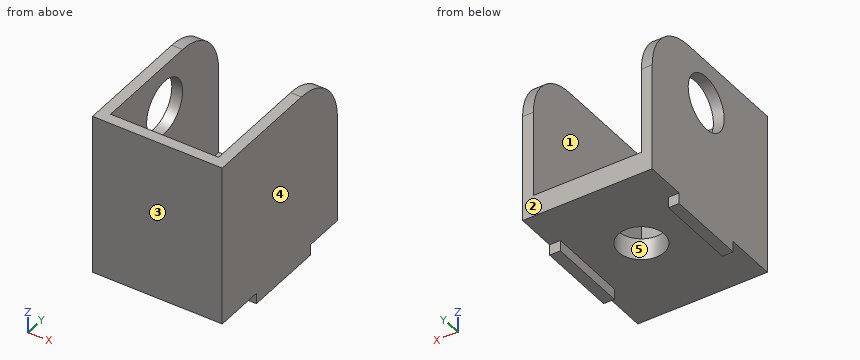
from build123d import *

# Parameters (mm, degrees)
SKETCH1_W           = 20
SKETCH1_H           = 30
SKETCH1_R           = 4.25
BOSS_EXTRUDE1_DEPTH = 4
SKETCH2_W           = 20
SKETCH2_H           = 30
BOSS_EXTRUDE2_DEPTH = 2
SKETCH4_R           = 5
BOSS_EXTRUDE3_DEPTH = 2
BOSS_EXTRUDE4_START = 2
BOSS_EXTRUDE4_DEPTH = 2
SKETCH6_W           = 2
SKETCH6_H           = 15
BOSS_EXTRUDE5_DEPTH = 2


with BuildPart() as part:
    # Sketch1 → Boss-Extrude1 (new body)
    with BuildSketch(Plane.XY):
        Rectangle(SKETCH1_W, SKETCH1_H)
        Circle(SKETCH1_R, mode=Mode.SUBTRACT)
    extrude(amount=BOSS_EXTRUDE1_DEPTH)

    # Sketch2 → Boss-Extrude2 (add)
    with BuildSketch(Plane(origin=(0, -15, 0), x_dir=(-1, 0, 0), z_dir=(0, -1, 0))):
        with Locations((0, -15)):
            Rectangle(SKETCH2_W, SKETCH2_H)
    extrude(amount=BOSS_EXTRUDE2_DEPTH)

    # Sketch4 → Boss-Extrude3 (add)
    with BuildSketch(Plane.ZY.offset(10)):
        with BuildLine():
            Line((0, 15), (20, 15))
            ThreePointArc((20, 15), (27.071067812, 12.071067812), (30, 5))
            Line((30, 5), (30, -17))
            Line((30, -17), (0, -17))
            Line((0, -17), (0, 15))
        make_face()
        with Locations((22, 0)):
            Circle(SKETCH4_R, mode=Mode.SUBTRACT)
    extrude(amount=BOSS_EXTRUDE3_DEPTH)

    # Sketch5 → Boss-Extrude4 (add)
    with BuildSketch(Plane(origin=(10, 0, 0), x_dir=(0, 0, -1), z_dir=(1, 0, 0)).offset(BOSS_EXTRUDE4_START)):
        with BuildLine():
            Line((0, 15), (-20, 15))
            ThreePointArc((-20, 15), (-27.071067812, 12.071067812), (-30, 5))
            Line((-30, 5), (-30, -17))
            Line((-30, -17), (0, -17))
            Line((0, -17), (0, 15))
        make_face()
    extrude(amount=-BOSS_EXTRUDE4_DEPTH)

    # Sketch6 → Boss-Extrude5 (add)
    with BuildSketch(Plane(origin=(0, 0, 0), x_dir=(-1, 0, 0), z_dir=(0, 0, -1))):
        with Locations((-11, 0)):
            Rectangle(SKETCH6_W, SKETCH6_H)
        with Locations((11, 0)):
            Rectangle(SKETCH6_W, SKETCH6_H)
    extrude(amount=BOSS_EXTRUDE5_DEPTH)


solid = part.part
The model under review builds one solid part; all positions refer to its coordinate system, in mm. Face numbers are marked on the shaded views. A direction names the side the tool comes from. Give positions to 0.01 mm unless a question says otherwise; leave off trailing zeros. Write each loop counter-clockwise with the first axis right and the second up, starting at its lowest first coordinate (ties: lowest second). Pieces come first, ordered by that corner, then holes. Notation, with made-up numbers: M -39.75,-26.5 L 13.25,-26.5 A7 ccw 13.25,-15.5 Z; hole C -12,30 d2. An arc over 180 degrees is marked long. One line per question, with ' | ' between items. Start each with the question number.
Item 1: We need section D-D on z = 26.5. Write out the cut boundary in (x, y), plus the area to 3 significant figures.
Item 2: We need section A-A on y = 0. Write out the cut boundary in (x, z), plus the area to 3 significant figures.
Item 3: We need section C-C on z = 12. Write out the cut boundary in (x, y).
Item 4: For the marked faces 1 and 2, list the 3-axis set-ups (+Z, -Z, +X, -X, +Y, -Y) from which the entire face can be reached by the end or side of a thin tool; tool diameter is ignored.
Item 5: Draft analysis for pull direction X (two halves, no side actions). For the marked faces 3, 4 and 5, state which applies: released by +X, released by -X, zero draft, split by the parting line, or undercut.
Item 6: For pin 1 (1 mm diameter, centred on x = 11.5, z = -1.5, fed in from -Y); pin 2 (12 mm diameter, centred on x = -4.5, z = 23.5, fed in from +Y); pin 3 (5 mm diameter, centred on x = -0.5, z = 8.5, fed in from +Y), all flat-tipped, find the tip position at first contact; note any pin that passes through.
Item 7: We need section B-B on x = 0.75. Write out the cut boundary in (y, z), plus the area to 3 significant figures.
Item 8: Wall thickness on line 1 (X direction, y = 2.5, z = 15.5); line 2 (Z direction, x = 7.25, y = -5); line 3 (Y direction, x = 0, z = 1.8): over which ranges is each line inside the solid? List them lowest first. Write a range as from..to.
Results found:
1) outline: M -12,-17 L 12,-17 L 12,12.6 L 10,12.6 L 10,-15 L -10,-15 L -10,-2.18 L -12,-2.18 Z; M -12,2.18 L -10,2.18 L -10,12.6 L -12,12.6 Z | area: 150 mm2
2) outline: M -12,-2 L -10,-2 L -10,0 L -4.25,0 L -4.25,4 L -10,4 L -10,17 L -12,17 Z; M -12,27 L -10,27 L -10,30 L -12,30 Z; M 4.25,0 L 10,0 L 10,-2 L 12,-2 L 12,30 L 10,30 L 10,4 L 4.25,4 Z | area: 154 mm2
3) outline: M -12,-17 L 12,-17 L 12,15 L 10,15 L 10,-15 L -10,-15 L -10,15 L -12,15 Z
4) face 1: +Z, +Y | face 2: +Z, -Z, +X, -X, +Y
5) face 3: zero draft | face 4: released by +X | face 5: undercut
6) pin 1: stops at y = -7.5 | pin 2: stops at y = 14.94 | pin 3: stops at y = -15
7) outline: M -17,0 L -4.18,0 L -4.18,4 L -15,4 L -15,30 L -17,30 Z; M 4.18,0 L 15,0 L 15,4 L 4.18,4 Z | area: 147 mm2
8) line 1: x = -12..-10, 10..12 | line 2: z = 0..4 | line 3: y = -17..-4.25, 4.25..15
